Geometry: final body of the model. Coordinates: model frame, mm. Round coordinates to 2 decimals unless told otherwise and drop trailing zeros. Loops run counter-clockwise (first coordinate to the right, second up) from the corner with the lowest first, then second, coordinate; pieces in that order, holes last. Notation, with made-up numbers: M 85,76.5 L 131,76.5 A27 cw 131,114.5 Z; hole C 39,-21.75 d9. An arc over 180 degrees is marked long. Return JSON: item names as keys, results as strings.
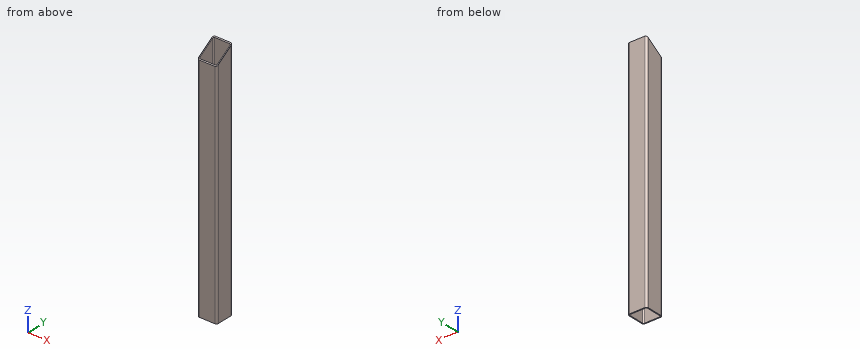
Autodesk Inventor part; units mm, degrees
ref_plane "Start plane" through (0, 0, 0) normal (0, 0, 1) x (1, 0, 0)
ref_plane "End plane" through (0, 0, 500) normal (0, 0, 1) x (1, 0, 0)
ref_plane "YZ Plane" through (0, 0, 0) normal (1, 0, 0) x (0, 1, 0)
ref_plane "Start plane" through (0, 0, 0) normal (0, 0, 1) x (1, 0, 0)
ref_plane "End plane" through (0, 0, 500) normal (0, 0, 1) x (1, 0, 0)
sketch "Sketch" plane through (0, 0, 0) normal (0, 0, 1) x (1, 0, 0)
  line L0 (-20, -16) -> (-20, 16)
  line L1 (-16, 20) -> (16, 20)
  line L2 (20, 16) -> (20, -16)
  line L3 (16, -20) -> (-16, -20)
  arc A0 (-20, -16) -> (-16, -20) centre (-16, -16) ccw
  arc A1 (20, 16) -> (16, 20) centre (16, 16) ccw
  arc A2 (-16, 20) -> (-20, 16) centre (-16, 16) ccw
  arc A3 (16, -20) -> (20, -16) centre (16, -16) ccw
  arc A4 (-16, 18) -> (-18, 16) centre (-16, 16) ccw
  line L4 (-16, 18) -> (16, 18)
  arc A5 (18, 16) -> (16, 18) centre (16, 16) ccw
  line L5 (18, 16) -> (18, -16)
  arc A6 (16, -18) -> (18, -16) centre (16, -16) ccw
  line L6 (16, -18) -> (-16, -18)
  arc A7 (-18, -16) -> (-16, -18) centre (-16, -16) ccw
  line L7 (-18, -16) -> (-18, 16)
  line L8 (0, 29.1598) -> (0, -29.1598) construction
  line L9 (-29.1598, 0) -> (29.1598, 0) construction
  dimension "d7" = 4
  dimension "d9" = 40
  dimension "d11" = 40
  dimension "d12" = 2
  dimension "d15" = 20
  dimension "d16" = 20
extrude "Body" add sketch "Sketch" along normal up to surface (500 mm away) from surface at 0
sketch "Sketch3" plane through (0, 0, 0) normal (0, 0, 1) x (1, 0, 0)
  line L0 (0, 0) -> (10, 0)
ref_plane "Work Plane3" through (0, 0, 0) normal (0, -1, 0) x (1, 0, 0)
sketch "Sketch5" plane through (0, 0, 0) normal (1, 0, 0) x (0, 1, 0)
  line L0 (-20, 0) -> (-20, 500)
  line L1 (-20, 0) -> (-20, 500)
  line L2 (20, 0) -> (20, 500)
  line L3 (20, 0) -> (20, 500)
  line L4 (-20, 500) -> (20, 500)
  line L5 (20, 500) -> (-20, 474.0237)
  point P0 (0, 0)
  point P1 (-20, 474.0237)
  dimension "d20" = 33
extrude "Extrusion2" cut sketch "Sketch5" along normal through all both and the other way through all
sketch "Sketch4" plane through (0, 0, 0) normal (0, -1, 0) x (1, 0, 0)
  line L0 (-2, 0) -> (12, 0)
  line L1 (-2, 500) -> (12, 500)
  dimension "d18" = 500
equation "\"d7\" = G_IR"
equation "\"d9\" = G_W"
equation "\"d11\" = G_H"
equation "\"d12\" = G_T"
equation "\"d15\" = 0.5 * d9"
equation "\"d16\" = 0.5 * d11"
equation "\"d3\" = G_L"
equation "\"G_W\" = 40"
equation "\"G_H\" = 40"
equation "\"G_T\" = 2"
equation "\"G_IR\" = 4"
equation "\"G_L\" = d18"
equation "\"G_OFFSET_START\" = 0"
equation "\"G_OFFSET_END\" = 0"
properties part number "ISO 4019 - 40x40x2 - 500" material "Steel, Mild"
Q1. Section query C-C (y = -7). Output: boundary loops of the cut face in (x, z), plus the area to 3 significant figures.
Determined:
{"outline": "M -20,0 L -18,0 L -18,482.47 L -20,482.47 Z; M 18,0 L 20,0 L 20,482.47 L 18,482.47 Z", "area": "1,930 mm^2"}
Q2. Section query B-B (z = 298.5). Output: boundary loops of the cut face in (x, y).
Determined:
{"outline": "M -20,-16 A4 ccw -16,-20 L 16,-20 A4 ccw 20,-16 L 20,16 A4 ccw 16,20 L -16,20 A4 ccw -20,16 Z; hole M -18,-16 A2 ccw -16,-18 L 16,-18 A2 ccw 18,-16 L 18,16 A2 ccw 16,18 L -16,18 A2 ccw -18,16 Z"}
Q3. Section query A-A (x = -3). Output: boundary loops of the cut face in (y, z), plus the area to 3 significant figures.
Determined:
{"outline": "M -20,0 L -18,0 L -18,475.32 L -20,474.02 Z; M 18,0 L 20,0 L 20,500 L 18,498.7 Z", "area": "1,950 mm^2"}
Q4. Material intervals for L1, parallel to Y at x = -2, z = 379.5; L2, parallel to X at y = 16.5, z = 297.5, sorted ascending.
Determined:
{"L1": "y = -20 to -18, 18 to 20", "L2": "x = -19.97 to -17.94, 17.94 to 19.97"}
Q5. Pin query (flat end, axial travel): pin 1 (12 mm diameter, centred on x = 7.5, y = 8, fed in from +Z). Return the tip coordinate at first contact, or that it passes through.
Determined:
{"pin 1": "passes through"}
